```python
from build123d import *

# Parameters (mm, degrees)
SKETCH1_W           = 59.999998659
SKETCH1_H           = 10.499999858
BOSS_EXTRUDE1_DEPTH = 3.000000026
CUT_EXTRUDE1_DEPTH  = 61.985652708
CUT_EXTRUDE2_DEPTH  = 61.944645671


with BuildPart() as part:
    # Sketch1 → Boss-Extrude1 (new body)
    with BuildSketch(Plane(origin=(0, 0, 0), x_dir=(-1, 0, 0), z_dir=(0, 0, -1))):
        with Locations((-29.99999933, 5.249999929)):
            Rectangle(SKETCH1_W, SKETCH1_H)
    extrude(amount=-BOSS_EXTRUDE1_DEPTH)

    # Sketch2 → Cut-Extrude1 (cut, through all)
    with BuildSketch(Plane.ZY):
        Polygon((3.000000026, 2.499999944), (3.000000026, 8.00000038), (2.499999944, 8.00000038), (2.499999944, 9.999999776), (1.000000047, 9.999999776), (1.000000047, 0.500000024), (2.499999944, 0.500000024), (2.499999944, 2.499999944), align=None)
    extrude(amount=-CUT_EXTRUDE1_DEPTH, mode=Mode.SUBTRACT)

    # Sketch3 → Cut-Extrude2 (cut, through all)
    with BuildSketch(Plane.XY.offset(1.000000047)):
        Polygon((30.559284613, 6.641833577), (30.316019431, 6.716332864), (30.063662678, 6.74864836), (29.809473082, 6.737850606), (29.560763389, 6.684250198), (29.324693605, 6.58938894), (29.108049348, 6.455995608), (28.917066753, 6.287908182), (28.757235035, 6.089962088), (28.633158654, 5.867851898), (28.548400849, 5.627966952), (28.505403548, 5.377208814), (28.505403548, 5.122791044), (28.548400849, 4.872032907), (28.633158654, 4.63214796), (28.757235035, 4.410037771), (28.917066753, 4.212091677), (29.108049348, 4.04400425), (29.324693605, 3.910611384), (29.560763389, 3.815749893), (29.809473082, 3.762149252), (30.063662678, 3.751351498), (30.316019431, 3.783667227), (30.559284613, 3.858166514), (30.786460266, 3.972706385), (30.991012231, 4.123991355), (31.167054549, 4.307670053), (31.309522688, 4.518457688), (31.414315104, 4.75029042), (31.478423625, 4.996498581), (31.500000507, 5.249999929), (31.478423625, 5.503501277), (31.414315104, 5.749709904), (31.309522688, 5.981542636), (31.167054549, 6.192329805), (30.991012231, 6.376008503), (30.786460266, 6.527293939), align=None)
    extrude(amount=-CUT_EXTRUDE2_DEPTH, mode=Mode.SUBTRACT)


solid = part.part
```
Geometry check sheet. Reference: the model listing, model coordinates, mm. A direction names the side the tool comes from. Round coordinates to 2 decimals unless told otherwise and drop trailing zeros. Loops run counter-clockwise (first coordinate to the right, second up) from the corner with the lowest first, then second, coordinate; pieces in that order, holes last. Notation, with made-up numbers: (-35, -13.5) - (-21, -13.5) arc R14 ccw to (-21, -5.5) - close; hole circle Ø1 at (64, 77.5). An arc over 180 degrees is marked (long way). Use a Markdown table: item, result.
Q1. Cross-section at A-A on z = 1.9. Record the cut outline in (x, y), plus the area to 3 significant figures.
Solutions:
| item | result |
|---|---|
| outline | (0, 0) - (60, 0) - (60, 0.5) - (0, 0.5) - close; (0, 10) - (60, 10) - (60, 10.5) - (0, 10.5) - close |
| area | 60.0 mm2 |
Q2. Cross-section at C-C on x = 42. Record the cut outline in (y, z).
Solutions:
| item | result |
|---|---|
| outline | (0, 0) - (10.5, 0) - (10.5, 3) - (8, 3) - (8, 2.5) - (10, 2.5) - (10, 1) - (0.5, 1) - (0.5, 2.5) - (2.5, 2.5) - (2.5, 3) - (0, 3) - close |
Q3. Material ranges on line 1 (Y direction, x = 33.5, z = 1.5); line 2 (Y direction, x = 53, z = 2.6); line 3 (Z direction, x = 37.5, y = 8.25), recorded low to high.
Solutions:
| item | result |
|---|---|
| line 1 | y = 0 to 0.5, 10 to 10.5 |
| line 2 | y = 0 to 2.5, 8 to 10.5 |
| line 3 | z = 0 to 1, 2.5 to 3 |
Q4. Access from +Z, -Z, +X, -X, +Y, -Y to the whole of each face (thin tool, end or side, straight path). Record for faces 1 (the flat face through (30, 9, 2.5)), 2 (the flat face through (0, 5.2, 0.8)).
Solutions:
| item | result |
|---|---|
| face 1 | +X, -X |
| face 2 | +Z, -Z, -X, +Y, -Y |
Q5. Draft check along Y on faces 3 (the flat face through (30, 10, 2)), 4 (the flat face through (30, 1, 3)), 5 (the flat face through (30, 0, 1)). Enter one of: released by +Y, released by -Y, zero draft, split by the parting line, or undercut.
Solutions:
| item | result |
|---|---|
| face 3 | undercut |
| face 4 | zero draft |
| face 5 | released by -Y |
Q6. Go/stop test with a flat-tipped pin: P1, Ø4, axis at x = 11.5, y = 5, coming from the +Z side. Record where the tip stops, or that it passes through.
Solutions:
| item | result |
|---|---|
| P1 | stops at z = 1 |
Q7. Cross-section at B-B on y = 9.5. Record the cut outline in (x, z), plus the area to 3 significant figures.
Solutions:
| item | result |
|---|---|
| outline | (0, 0) - (60, 0) - (60, 1) - (0, 1) - close; (0, 2.5) - (60, 2.5) - (60, 3) - (0, 3) - close |
| area | 90.0 mm2 |
Q8. Cross-section at D-D on y = 3. Record the cut outline in (x, z).
Solutions:
| item | result |
|---|---|
| outline | (0, 0) - (60, 0) - (60, 1) - (0, 1) - close |
